The listing builds one solid part. Answer for the finished solid, in the listing's coordinates (mm). Round coordinates to 2 decimals unless told otherwise and drop trailing zeros. Loops run counter-clockwise (first coordinate to the right, second up) from the corner with the lowest first, then second, coordinate; pieces in that order, holes last. Notation, with made-up numbers: (18, 0) -> (28, 0) arc R20 ccw to (28, 13) -> close; hole circle Ø2 at (33.25, -17.75). An arc over 180 degrees is marked (long way). Write each question's results on one line, items separated by ' | '. Start each with the question number.
(1) The part is cut by section A-A (y = 56.5). Determine the outline of the cut face in (x, z), plus the area to 3 significant figures.
(2) The part is cut by section C-C (x = 54). Determine the outline of the cut face in (y, z), plus the area to 3 significant figures.
(3) The part is cut by section D-D (z = 0.4). Count the separate pieces of the cut face and the enclosed holes in it, plus the area to 3 significant figures.
(4) Flat-ended cylindrical pins translate along their axes: pin 1 (2 mm diameter, centred on x = 40, y = 13.5, fed in from -Z); pin 2 (0.6 mm diameter, centred on x = 3, z = 1, fed in from +Y); pin 3 (5 mm diameter, centred on x = 60, y = -57.75, fed in from +Z); pin 4 (1 mm diameter, centred on y = -29, z = 1, fed in from -X). Find the tip coordinate at first contact, or state that the pin passes through.
(5) Straight lines are drawn through the part: probe 1 along Y at (x, z) = (6.5, 1.5); probe 2 along Y at (x, z) = (60, 0.9); probe 3 along Y at (x, z) = (-62, 1.45). For each, find the intervals that lie inside material, in ascending order.
(6) The part is cut by section B-B (x = -60). Determine the outline of the cut face in (y, z).
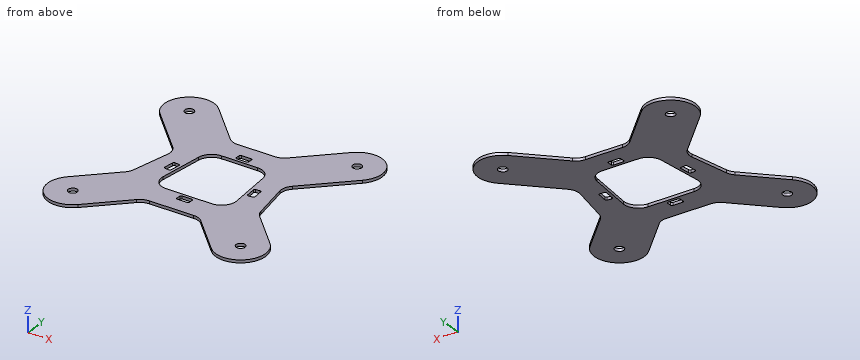
```python
from build123d import *

# Parameters (mm, degrees)
AUFSATZ_LINEAR_AUSTRAGEN1_DEPTH      = 2
SKIZZE2_R                            = 3.2
SCHNITT_LINEAR_AUSTRAGEN1_DEPTH      = 2
SCHNITT_LINEAR_AUSTRAGEN3_DEPTH      = 2
VERRUNDUNG1_R                        = 10
VERRUNDUNG2_R                        = 10
SCHNITT_LINEAR_AUSTRAGEN4_DEPTH      = 112.222811939
SCHNITT_LINEAR_AUSTRAGEN4_DEPTH_BACK = 112.222811939


with BuildPart() as part:
    # Skizze1 → Aufsatz-Linear austragen1 (new body)
    with BuildSketch(Plane.XY):
        with BuildLine():
            Line((17.5, 44.5), (-17.5, 44.5))
            Line((-17.5, 44.5), (-47.625631329, 74.625631329))
            ThreePointArc((-47.625631329, 74.625631329), (-72.374368671, 74.625631329), (-72.374368671, 49.876893988))
            Line((-72.374368671, 49.876893988), (-39, 16.502525317))
            Line((-39, 16.502525317), (-46, -19))
            Line((-46, -19), (-72.374368671, -45.374368671))
            ThreePointArc((-72.374368671, -45.374368671), (-72.374368671, -70.123106012), (-47.625631329, -70.123106012))
            Line((-47.625631329, -70.123106012), (-20, -42.497474683))
            Line((-20, -42.497474683), (20, -42.497474683))
            Line((20, -42.497474683), (47.625631329, -70.123106012))
            ThreePointArc((47.625631329, -70.123106012), (72.374368671, -70.123106012), (72.374368671, -45.374368671))
            Line((72.374368671, -45.374368671), (46, -19))
            Line((46, -19), (39, 16.502525317))
            Line((39, 16.502525317), (72.374368671, 49.876893988))
            ThreePointArc((72.374368671, 49.876893988), (72.374368671, 74.625631329), (47.625631329, 74.625631329))
            Line((47.625631329, 74.625631329), (17.5, 44.5))
        make_face()
    extrude(amount=AUFSATZ_LINEAR_AUSTRAGEN1_DEPTH)

    # Skizze2 → Schnitt-Linear austragen1 (cut)
    with BuildSketch(Plane.XY.offset(2)):
        with Locations((-60, -57.748737342)):
            Circle(SKIZZE2_R)
        with Locations((-60, 62.251262658)):
            Circle(SKIZZE2_R)
        with Locations((60, -57.748737342)):
            Circle(SKIZZE2_R)
        with Locations((60, 62.251262658)):
            Circle(SKIZZE2_R)
    extrude(amount=-SCHNITT_LINEAR_AUSTRAGEN1_DEPTH, mode=Mode.SUBTRACT)

    # Skizze4 → Schnitt-Linear austragen3 (cut)
    with BuildSketch(Plane.XY.offset(2)):
        Polygon((-22, 27.5), (22, 27.5), (27.5, -24.5), (-27.5, -24.5), align=None)
    extrude(amount=-SCHNITT_LINEAR_AUSTRAGEN3_DEPTH, mode=Mode.SUBTRACT)

    # Verrundung1
    verrundung1_edges = [part.edges().sort_by_distance(p)[0] for p in [
        (-27.5, -24.5, 1),
        (-22, 27.5, 1),
        (22, 27.5, 1),
        (27.5, -24.5, 1),
    ]]
    fillet(verrundung1_edges, radius=VERRUNDUNG1_R)

    # Verrundung2
    verrundung2_edges = [part.edges().sort_by_distance(p)[0] for p in [
        (-17.5, 44.5, 1),
        (17.5, 44.5, 1),
        (39, 16.502525317, 1),
        (46, -19, 1),
        (20, -42.497474683, 1),
        (-20, -42.497474683, 1),
        (-46, -19, 1),
        (-39, 16.502525317, 1),
    ]]
    fillet(verrundung2_edges, radius=VERRUNDUNG2_R)

    # Skizze5 → Schnitt-Linear austragen4 (cut, two sides: drawn at the far end of the back side and taken through both)
    with BuildSketch(Plane.XY.offset(2).offset(-SCHNITT_LINEAR_AUSTRAGEN4_DEPTH_BACK)):
        with BuildLine():
            Line((-3.5, 34.5), (3.5, 34.5))
            ThreePointArc((3.5, 34.5), (4.207106781, 34.207106781), (4.5, 33.5))
            Line((4.5, 33.5), (4.5, 30.5))
            ThreePointArc((4.5, 30.5), (4.207106781, 29.792893219), (3.5, 29.5))
            Line((3.5, 29.5), (-3.5, 29.5))
            ThreePointArc((-3.5, 29.5), (-4.207106781, 29.792893219), (-4.5, 30.5))
            Line((-4.5, 30.5), (-4.5, 33.5))
            ThreePointArc((-4.5, 33.5), (-4.207106781, 34.207106781), (-3.5, 34.5))
        make_face()
        with BuildLine():
            Line((-30.424300248, 4.895768288), (-27.440941448, 4.580220723))
            ThreePointArc((-27.440941448, 4.580220723), (-26.768564282, 4.214576928), (-26.551671036, 3.480585268))
            Line((-26.551671036, 3.480585268), (-27.287948689, -3.480585268))
            ThreePointArc((-27.287948689, -3.480585268), (-27.653592484, -4.152962433), (-28.387584144, -4.369855679))
            Line((-28.387584144, -4.369855679), (-31.370942945, -4.054308114))
            ThreePointArc((-31.370942945, -4.054308114), (-32.04332011, -3.688664319), (-32.260213356, -2.954672658))
            Line((-32.260213356, -2.954672658), (-31.523935704, 4.006497877))
            ThreePointArc((-31.523935704, 4.006497877), (-31.158291909, 4.678875042), (-30.424300248, 4.895768288))
        make_face()
        with BuildLine():
            Line((26.551671036, 3.480585268), (27.287948689, -3.480585268))
            ThreePointArc((27.287948689, -3.480585268), (27.653592484, -4.152962433), (28.387584144, -4.369855679))
            Line((28.387584144, -4.369855679), (31.370942945, -4.054308114))
            ThreePointArc((31.370942945, -4.054308114), (32.04332011, -3.688664319), (32.260213356, -2.954672658))
            Line((32.260213356, -2.954672658), (31.523935704, 4.006497877))
            ThreePointArc((31.523935704, 4.006497877), (31.158291909, 4.678875042), (30.424300248, 4.895768288))
            Line((30.424300248, 4.895768288), (27.440941448, 4.580220723))
            ThreePointArc((27.440941448, 4.580220723), (26.768564282, 4.214576928), (26.551671036, 3.480585268))
        make_face()
        with BuildLine():
            Line((4.5, -30.5), (4.5, -27.5))
            ThreePointArc((4.5, -27.5), (4.207106781, -26.792893219), (3.5, -26.5))
            Line((3.5, -26.5), (-3.5, -26.5))
            ThreePointArc((-3.5, -26.5), (-4.207106781, -26.792893219), (-4.5, -27.5))
            Line((-4.5, -27.5), (-4.5, -30.5))
            ThreePointArc((-4.5, -30.5), (-4.207106781, -31.207106781), (-3.5, -31.5))
            Line((-3.5, -31.5), (3.5, -31.5))
            ThreePointArc((3.5, -31.5), (4.207106781, -31.207106781), (4.5, -30.5))
        make_face()
    extrude(amount=SCHNITT_LINEAR_AUSTRAGEN4_DEPTH + SCHNITT_LINEAR_AUSTRAGEN4_DEPTH_BACK, mode=Mode.SUBTRACT)


solid = part.part
```
Checked values:
1) outline: (-76.53, 0) -> (-29.5, 0) -> (-29.5, 2) -> (-76.53, 2) -> close; (29.5, 0) -> (76.53, 0) -> (76.53, 2) -> (29.5, 2) -> close | area: 188 mm2
2) outline: (-74.19, 0) -> (-27, 0) -> (-27, 2) -> (-74.19, 2) -> close; (31.5, 0) -> (78.69, 0) -> (78.69, 2) -> (31.5, 2) -> close | area: 189 mm2
3) separate pieces: 1 | enclosed holes: 9 | area: 11,100 mm2
4) pin 1: stops at z = 0 | pin 2: stops at y = 44.5 | pin 3: passes through | pin 4: stops at x = -56.5
5) probe 1: y = -42.5 to -24.5, 27.5 to 44.5 | probe 2: y = -75.25 to -60.95, -54.55 to -33, 37.5 to 59.05, 65.45 to 79.75 | probe 3: y = -75.13 to -60.25, -55.25 to -35, 39.5 to 59.75, 64.75 to 79.64
6) outline: (-75.25, 0) -> (-60.95, 0) -> (-60.95, 2) -> (-75.25, 2) -> close; (-54.55, 0) -> (-33, 0) -> (-33, 2) -> (-54.55, 2) -> close; (37.5, 0) -> (59.05, 0) -> (59.05, 2) -> (37.5, 2) -> close; (65.45, 0) -> (79.75, 0) -> (79.75, 2) -> (65.45, 2) -> close
